from build123d import *

# Parameters (mm, degrees)
SKETCH086_W             = 8.6
SKETCH086_H             = 20
PAD067_DEPTH            = 5
SKETCH087_W             = 8.6
SKETCH087_H             = 20
PAD068_DEPTH            = 5
BODY068_PLACEMENT_ANGLE = 334.29
SKETCH088_W             = 8.6
SKETCH088_H             = 20
PAD069_DEPTH            = 5
BODY069_PLACEMENT_ANGLE = 308.58
SKETCH089_W             = 8.6
SKETCH089_H             = 20
PAD070_DEPTH            = 5
BODY070_PLACEMENT_ANGLE = 282.87
SKETCH090_W             = 8.6
SKETCH090_H             = 20
PAD071_DEPTH            = 5
BODY071_PLACEMENT_ANGLE = 257.16
SKETCH091_W             = 8.6
SKETCH091_H             = 20
PAD072_DEPTH            = 5
BODY072_PLACEMENT_ANGLE = 231.45
SKETCH092_W             = 8.6
SKETCH092_H             = 20
PAD073_DEPTH            = 5
BODY073_PLACEMENT_ANGLE = 205.74
SKETCH093_W             = 8.6
SKETCH093_H             = 20
PAD074_DEPTH            = 5
BODY074_PLACEMENT_ANGLE = 179.97
SKETCH094_W             = 8.6
SKETCH094_H             = 20
PAD075_DEPTH            = 5
BODY075_PLACEMENT_ANGLE = 154.26
SKETCH095_W             = 8.6
SKETCH095_H             = 20
PAD076_DEPTH            = 5
BODY076_PLACEMENT_ANGLE = 128.55
SKETCH096_W             = 8.6
SKETCH096_H             = 20
PAD077_DEPTH            = 5
BODY077_PLACEMENT_ANGLE = 102.84
SKETCH097_W             = 8.6
SKETCH097_H             = 20
PAD078_DEPTH            = 5
BODY078_PLACEMENT_ANGLE = 77.13
SKETCH098_W             = 8.6
SKETCH098_H             = 20
PAD079_DEPTH            = 5
BODY079_PLACEMENT_ANGLE = 51.42
SKETCH099_W             = 8.6
SKETCH099_H             = 20
PAD080_DEPTH            = 5
BODY080_PLACEMENT_ANGLE = 25.71
SKETCH019_R             = 42
SKETCH019_R_2           = 1.5
PAD016_DEPTH            = 8
SKETCH100_R             = 8.75
POCKET009_DEPTH         = 1


with BuildPart() as body067:
    # Sketch086 → Pad067 (new body)
    with BuildSketch(Plane.YZ):
        with Locations((0, 31.5)):
            Rectangle(SKETCH086_W, SKETCH086_H)
    extrude(amount=PAD067_DEPTH)


with BuildPart() as body068:
    # Sketch087 → Pad068 (new body)
    with BuildSketch(Plane.YZ):
        with Locations((0, 31.5)):
            Rectangle(SKETCH087_W, SKETCH087_H)
    extrude(amount=PAD068_DEPTH)


with BuildPart() as body068_1:
    # Body068 placement: moved
    add(body068.part.rotate(Axis((0, 0, 0), (1, 0, 0)), BODY068_PLACEMENT_ANGLE))


with BuildPart() as body069:
    # Sketch088 → Pad069 (new body)
    with BuildSketch(Plane.YZ):
        with Locations((0, 31.5)):
            Rectangle(SKETCH088_W, SKETCH088_H)
    extrude(amount=PAD069_DEPTH)


with BuildPart() as body069_1:
    # Body069 placement: moved
    add(body069.part.rotate(Axis((0, 0, 0), (1, 0, 0)), BODY069_PLACEMENT_ANGLE))


with BuildPart() as body070:
    # Sketch089 → Pad070 (new body)
    with BuildSketch(Plane.YZ):
        with Locations((0, 31.5)):
            Rectangle(SKETCH089_W, SKETCH089_H)
    extrude(amount=PAD070_DEPTH)


with BuildPart() as body070_1:
    # Body070 placement: moved
    add(body070.part.rotate(Axis((0, 0, 0), (1, 0, 0)), BODY070_PLACEMENT_ANGLE))


with BuildPart() as body071:
    # Sketch090 → Pad071 (new body)
    with BuildSketch(Plane.YZ):
        with Locations((0, 31.5)):
            Rectangle(SKETCH090_W, SKETCH090_H)
    extrude(amount=PAD071_DEPTH)


with BuildPart() as body071_1:
    # Body071 placement: moved
    add(body071.part.rotate(Axis((0, 0, 0), (1, 0, 0)), BODY071_PLACEMENT_ANGLE))


with BuildPart() as body072:
    # Sketch091 → Pad072 (new body)
    with BuildSketch(Plane.YZ):
        with Locations((0, 31.5)):
            Rectangle(SKETCH091_W, SKETCH091_H)
    extrude(amount=PAD072_DEPTH)


with BuildPart() as body072_1:
    # Body072 placement: moved
    add(body072.part.rotate(Axis((0, 0, 0), (1, 0, 0)), BODY072_PLACEMENT_ANGLE))


with BuildPart() as body073:
    # Sketch092 → Pad073 (new body)
    with BuildSketch(Plane.YZ):
        with Locations((0, 31.5)):
            Rectangle(SKETCH092_W, SKETCH092_H)
    extrude(amount=PAD073_DEPTH)


with BuildPart() as body073_1:
    # Body073 placement: moved
    add(body073.part.rotate(Axis((0, 0, 0), (1, 0, 0)), BODY073_PLACEMENT_ANGLE))


with BuildPart() as body074:
    # Sketch093 → Pad074 (new body)
    with BuildSketch(Plane.YZ):
        with Locations((0, 31.5)):
            Rectangle(SKETCH093_W, SKETCH093_H)
    extrude(amount=PAD074_DEPTH)


with BuildPart() as body074_1:
    # Body074 placement: moved
    add(body074.part.rotate(Axis((0, 0, 0), (1, 0, 0)), BODY074_PLACEMENT_ANGLE))


with BuildPart() as body075:
    # Sketch094 → Pad075 (new body)
    with BuildSketch(Plane.YZ):
        with Locations((0, 31.5)):
            Rectangle(SKETCH094_W, SKETCH094_H)
    extrude(amount=PAD075_DEPTH)


with BuildPart() as body075_1:
    # Body075 placement: moved
    add(body075.part.rotate(Axis((0, 0, 0), (1, 0, 0)), BODY075_PLACEMENT_ANGLE))


with BuildPart() as body076:
    # Sketch095 → Pad076 (new body)
    with BuildSketch(Plane.YZ):
        with Locations((0, 31.5)):
            Rectangle(SKETCH095_W, SKETCH095_H)
    extrude(amount=PAD076_DEPTH)


with BuildPart() as body076_1:
    # Body076 placement: moved
    add(body076.part.rotate(Axis((0, 0, 0), (1, 0, 0)), BODY076_PLACEMENT_ANGLE))


with BuildPart() as body077:
    # Sketch096 → Pad077 (new body)
    with BuildSketch(Plane.YZ):
        with Locations((0, 31.5)):
            Rectangle(SKETCH096_W, SKETCH096_H)
    extrude(amount=PAD077_DEPTH)


with BuildPart() as body077_1:
    # Body077 placement: moved
    add(body077.part.rotate(Axis((0, 0, 0), (1, 0, 0)), BODY077_PLACEMENT_ANGLE))


with BuildPart() as body078:
    # Sketch097 → Pad078 (new body)
    with BuildSketch(Plane.YZ):
        with Locations((0, 31.5)):
            Rectangle(SKETCH097_W, SKETCH097_H)
    extrude(amount=PAD078_DEPTH)


with BuildPart() as body078_1:
    # Body078 placement: moved
    add(body078.part.rotate(Axis((0, 0, 0), (1, 0, 0)), BODY078_PLACEMENT_ANGLE))


with BuildPart() as body079:
    # Sketch098 → Pad079 (new body)
    with BuildSketch(Plane.YZ):
        with Locations((0, 31.5)):
            Rectangle(SKETCH098_W, SKETCH098_H)
    extrude(amount=PAD079_DEPTH)


with BuildPart() as body079_1:
    # Body079 placement: moved
    add(body079.part.rotate(Axis((0, 0, 0), (1, 0, 0)), BODY079_PLACEMENT_ANGLE))


with BuildPart() as body080:
    # Sketch099 → Pad080 (new body)
    with BuildSketch(Plane.YZ):
        with Locations((0, 31.5)):
            Rectangle(SKETCH099_W, SKETCH099_H)
    extrude(amount=PAD080_DEPTH)


with BuildPart() as body080_1:
    # Body080 placement: moved
    add(body080.part.rotate(Axis((0, 0, 0), (1, 0, 0)), BODY080_PLACEMENT_ANGLE))


with BuildPart() as body016:
    # Sketch019 → Pad016 (new body)
    with BuildSketch(Plane.YZ):
        Circle(SKETCH019_R)
        with Locations((0, 5)):
            Circle(SKETCH019_R_2, mode=Mode.SUBTRACT)
        with Locations((4.330127, -2.5)):
            Circle(SKETCH019_R_2, mode=Mode.SUBTRACT)
        with Locations((-4.330127, -2.5)):
            Circle(SKETCH019_R_2, mode=Mode.SUBTRACT)
    extrude(amount=PAD016_DEPTH)

    # Boolean014: cut Body067, Body068, Body069, Body070, Body071, Body072, Body073, Body074, Body075, Body076, Body077, Body078, Body079, Body080
    add(body067.part, mode=Mode.SUBTRACT)
    add(body068_1.part, mode=Mode.SUBTRACT)
    add(body069_1.part, mode=Mode.SUBTRACT)
    add(body070_1.part, mode=Mode.SUBTRACT)
    add(body071_1.part, mode=Mode.SUBTRACT)
    add(body072_1.part, mode=Mode.SUBTRACT)
    add(body073_1.part, mode=Mode.SUBTRACT)
    add(body074_1.part, mode=Mode.SUBTRACT)
    add(body075_1.part, mode=Mode.SUBTRACT)
    add(body076_1.part, mode=Mode.SUBTRACT)
    add(body077_1.part, mode=Mode.SUBTRACT)
    add(body078_1.part, mode=Mode.SUBTRACT)
    add(body079_1.part, mode=Mode.SUBTRACT)
    add(body080_1.part, mode=Mode.SUBTRACT)

    # Sketch100 (on DatumPlane) → Pocket009 (cut)
    with BuildSketch(Plane(origin=(0, 0, 0), x_dir=(0, -1, 0), z_dir=(-1, 0, 0))):
        Circle(SKETCH100_R)
    extrude(amount=-POCKET009_DEPTH, mode=Mode.SUBTRACT)


solid = body016.part
Can you work these out from the model? Positions are in its coordinate system, mm. Give positions to 0.01 mm unless a question says otherwise; leave off trailing zeros. Loops run counter-clockwise (first coordinate to the right, second up) from the corner with the lowest first, then second, coordinate; pieces in that order, holes last. Notation, with made-up numbers: (70, -40) -> (112, -40) arc R29 cw to (112, -12) -> close; hole circle Ø2 at (-5, -25). An arc over 180 degrees is marked (long way). Write item = value, one per line.
1) Suppose I cut it at A-A on y = 0. Write out the boundary of the cut face in (x, z), then the cut area to 4 significant figures.
Check result:
outline = (0, -42) -> (8, -42) -> (8, 3.5) -> (1, 3.5) -> (1, -8.75) -> (0, -8.75) -> (0, -21.5) -> (5, -21.5) -> (5, -41.5) -> (0, -41.5) -> close; (0, 8.75) -> (1, 8.75) -> (1, 6.5) -> (8, 6.5) -> (8, 42) -> (0, 42) -> (0, 41.5) -> (5, 41.5) -> (5, 21.5) -> (0, 21.5) -> close
area = 433.5 mm2
2) Will these pins go through, and if not, where does the flat tip stop? pin 1 (2.5 mm diameter, centred on x = 2, z = 28.5, fed in from +Y); pin 2 (3 mm diameter, centred on x = 4, y = -24.5, fed in from -Z); pin 3 (3 mm diameter, centred on x = 1, z = -10, fed in from +Y); pin 4 (1.8 mm diameter, centred on y = -4.33, z = -2.5, fed in from +X).
Check result:
pin_1 = 31.96
pin_2 = -35.14
pin_3 = 41.13
pin_4 = through
3) Suppose I cut it at C-C on z = 24.5. Write out the boundary of the cut face in (x, y).
Check result:
outline = (0, -34.11) -> (8, -34.11) -> (8, 34.11) -> (0, 34.11) -> (0, 33.54) -> (5, 33.54) -> (5, 23.82) -> (0, 23.82) -> (0, 16.57) -> (5, 16.57) -> (5, 7.02) -> (0, 7.02) -> (0, 4.3) -> (5, 4.3) -> (5, -4.3) -> (0, -4.3) -> (0, -7.02) -> (5, -7.02) -> (5, -16.57) -> (0, -16.57) -> (0, -23.82) -> (5, -23.82) -> (5, -33.54) -> (0, -33.54) -> close
4) Suppose I cut it at B-B on z = -2.5. Write out the boundary of the cut face in (x, y), then the cut area to 3 significant figures.
Check result:
outline = (0, -41.93) -> (8, -41.93) -> (8, -5.83) -> (1, -5.83) -> (1, -8.39) -> (0, -8.39) -> (0, -21.48) -> (5, -21.48) -> (5, -30.32) -> (0, -30.32) -> close; (0, 8.39) -> (1, 8.39) -> (1, 5.83) -> (8, 5.83) -> (8, 41.93) -> (0, 41.93) -> (0, 30.32) -> (5, 30.32) -> (5, 21.48) -> (0, 21.48) -> close; (1, -2.83) -> (8, -2.83) -> (8, 2.83) -> (1, 2.83) -> close
area = 524 mm2
5) I need wall thicknesses on L1, parallel to Z at x = 0.65, y = 0; L2, parallel to Z at x = 1.5, y = 0; L3, parallel to Z at x = 2.5, y = -11. Which ranges of each line are inside material? Lowest first, please. Write a range as from..to.
Check result:
L1 = -42..-41.5, -21.5..-8.75, 8.75..21.5, 41.5..42
L2 = -42..-41.5, -21.5..3.5, 6.5..21.5, 41.5..42
L3 = -40.53..-32.72, -18.56..18.57, 32.76..40.53
6) Suppose I cut it at D-D on x = 2. Give the number of separate pieces and of enclosed holes in the cut face, then the cut area to 3 significant figures.
Check result:
separate_pieces = 1
enclosed_holes = 17
area = 3,110 mm2
